from build123d import *

# Parameters (mm, degrees)
ESBO_O1_R                = 60
ESBO_O1_R_2              = 3
RESSALTO_EXTRUS_O4_DEPTH = 30
ESBO_O6_R                = 60
ESBO_O6_R_2              = 5
RESSALTO_EXTRUS_O8_DEPTH = 30
ESBO_O9_R                = 60
CORTE_EXTRUS_O1_DEPTH    = 91
ESBO_O11_W               = 62
ESBO_O11_H               = 15
CORTE_EXTRUS_O2_DEPTH    = 60.514704065
ESBO_O12_R               = 2.5
CORTE_EXTRUS_O3_DEPTH    = 15
ESBO_O15_R               = 3
RESSALTO_EXTRUS_O9_DEPTH = 5
ESBO_O16_R               = 4.75
CORTE_EXTRUS_O4_DEPTH    = 6


with BuildPart() as part:
    # Esboço1 → Ressalto-extrusão4 (new body)
    with BuildSketch(Plane.XY):
        Circle(ESBO_O1_R)
        with Locations((-14.142135624, 14.142135624)):
            Circle(ESBO_O1_R_2, mode=Mode.SUBTRACT)
        with Locations((14.142135624, 14.142135624)):
            Circle(ESBO_O1_R_2, mode=Mode.SUBTRACT)
        with Locations((14.142135624, -14.142135624)):
            Circle(ESBO_O1_R_2, mode=Mode.SUBTRACT)
        with Locations((-14.142135624, -14.142135624)):
            Circle(ESBO_O1_R_2, mode=Mode.SUBTRACT)
        with Locations((0, 20)):
            Circle(ESBO_O1_R_2, mode=Mode.SUBTRACT)
    extrude(amount=-RESSALTO_EXTRUS_O4_DEPTH)

    # Esboço6 → Ressalto-extrusão8 (add)
    with BuildSketch(Plane.XY):
        Circle(ESBO_O6_R)
        with Locations((-14.142135624, -14.142135624)):
            Circle(ESBO_O6_R_2, mode=Mode.SUBTRACT)
        with Locations((14.142135624, -14.142135624)):
            Circle(ESBO_O6_R_2, mode=Mode.SUBTRACT)
        with Locations((-14.142135624, 14.142135624)):
            Circle(ESBO_O6_R_2, mode=Mode.SUBTRACT)
        with Locations((14.142135624, 14.142135624)):
            Circle(ESBO_O6_R_2, mode=Mode.SUBTRACT)
    extrude(amount=-RESSALTO_EXTRUS_O8_DEPTH)

    # Esboço9 → Corte-extrusão1 (cut, through all)
    with BuildSketch(Plane(origin=(0, 0, -30), x_dir=(-1, 0, 0), z_dir=(0, 0, -1))):
        Circle(ESBO_O9_R)
        Polygon((-31, 30), (0, 30), (31, 30), (31, 0), (31, -31), (31, -41), (-31, -41), (-31, -31), (-31, 0), align=None, mode=Mode.SUBTRACT)
    extrude(amount=-CORTE_EXTRUS_O1_DEPTH, mode=Mode.SUBTRACT)

    # Esboço11 → Corte-extrusão2 (cut, through all)
    with BuildSketch(Plane.XY):
        with Locations((0, -33.5)):
            Rectangle(ESBO_O11_W, ESBO_O11_H)
    extrude(amount=-CORTE_EXTRUS_O2_DEPTH, mode=Mode.SUBTRACT)

    # Esboço12 → Corte-extrusão3 (cut)
    with BuildSketch(Plane.XZ.offset(26)):
        with Locations(Location((24.07, -15, 0), (0, 0, 270))):
            Circle(ESBO_O12_R)
        with Locations(Location((0, -15, 0), (0, 0, 270))):
            Circle(ESBO_O12_R)
        with Locations(Location((-24.07, -15, 0), (0, 0, 270))):
            Circle(ESBO_O12_R)
    extrude(amount=-CORTE_EXTRUS_O3_DEPTH, mode=Mode.SUBTRACT)

    # Esboço15 → Ressalto-extrusão9 (add)
    with BuildSketch(Plane.XY):
        with Locations((0, 20)):
            Circle(ESBO_O15_R)
    extrude(amount=RESSALTO_EXTRUS_O9_DEPTH)

    # Esboço16 → Corte-extrusão4 (cut)
    with BuildSketch(Plane(origin=(0, 0, -30), x_dir=(-1, 0, 0), z_dir=(0, 0, -1))):
        with Locations((14.142135624, 14.142135624)):
            Circle(ESBO_O16_R)
        with Locations((14.142135624, -14.142135624)):
            Circle(ESBO_O16_R)
        with Locations((-14.142135624, 14.142135624)):
            Circle(ESBO_O16_R)
        with Locations((-14.142135624, -14.142135624)):
            Circle(ESBO_O16_R)
    extrude(amount=-CORTE_EXTRUS_O4_DEPTH, mode=Mode.SUBTRACT)


solid = part.part
Input: part model. Units: mm. Frame: model coordinates. A direction names the side the tool comes from. Give positions to 0.01 mm unless a question says otherwise; leave off trailing zeros. Loops run counter-clockwise (first coordinate to the right, second up) from the corner with the lowest first, then second, coordinate; pieces in that order, holes last. Notation, with made-up numbers: M -25,41.5 L -5,41.5 A20 ccw -5,65.5 Z; hole C -37,13.5 d8. An arc over 180 degrees is marked long. Use one line per item in the form item = value.
1. Pull-direction query (Z, two-part tool) for faces 1 (the face through (13.2, -17.2, -24)), 2 (the face through (0, 2, 0)), 3 (the face through (-24, -11, -15)), 4 (the face through (9.61, -12.72, -27.04)); classes: released by +Z, released by -Z, zero draft, split by the parting line, or undercut.
Numbers:
face_1 = released by -Z
face_2 = released by +Z
face_3 = undercut
face_4 = zero draft
2. Line query: L1, parallel to X at y = 14, z = -27.5; L2, parallel to Y at x = -11.5, z = -12.5; L3, parallel to Y at x = -10, z = -27.5. Output: solid intervals per line, ascending.
Numbers:
L1 = -31 to -18.89, -9.39 to 9.39, 18.89 to 31
L2 = -26 to -15.56, -12.72 to 12.72, 15.56 to 30
L3 = -26 to -16.47, -11.82 to 11.82, 16.47 to 30
3. Section query D-D, the plane x = -14. Return the cut outline in (y, z), and give its area (3 significant figures).
Numbers:
outline = M -26,-30 L -18.89,-30 L -18.89,-24 L -17.14,-24 L -17.14,0 L -26,0 Z; M -11.15,-24 L -9.39,-24 L -9.39,-30 L 9.39,-30 L 9.39,-24 L 11.15,-24 L 11.15,0 L -11.15,0 Z; M 17.14,-24 L 18.89,-24 L 18.89,-30 L 30,-30 L 30,0 L 17.14,0 Z
area = 1,280 mm²
4. Reachability of faces 5 (the face through (0, 2, -30)), 6 (the face through (-25.591, -18.605, -13.016)), 7 (the face through (-10.64, 17.35, -27.04)) from +Z, -Z, +X, -X, +Y, -Y: full face, straight path, thin tool, end or side. Return the list, or none.
Numbers:
face_5 = -Z, +X, -X, +Y, -Y
face_6 = -Y
face_7 = -Z
5. Section query C-C, the plane z = -9. Return the cut outline in (x, y).
Numbers:
outline = M -31,-26 L 31,-26 L 31,30 L -31,30 Z; hole C -14.14,-14.14 d6; hole C -14.14,14.14 d6; hole C 14.14,-14.14 d6; hole C 14.14,14.14 d6
6. First-contact query: pin 1 (5 mm diameter, centred on x = 14.14, y = 14.14, fed in from -Z); pin 2 (7 mm diameter, centred on x = 14.14, y = -14.14, fed in from -Z); pin 3 (10 mm diameter, centred on x = -2.5, y = -10.5, fed in from +Z). Flat tips, straight axial feed; report the tip coordinate or a pass-through.
Numbers:
pin_1 = through
pin_2 = -24
pin_3 = 0
7. Section query A-A, the plane x = 24.07. Return the cut outline in (y, z).
Numbers:
outline = M -26,-30 L 30,-30 L 30,0 L -26,0 L -26,-12.5 L -11,-12.5 L -11,-17.5 L -26,-17.5 Z
8. Section query B-B, the plane y = 20. Return the cut outline in (x, z).
Numbers:
outline = M -31,-30 L 31,-30 L 31,0 L 3,0 L 3,5 L -3,5 L -3,0 L -31,0 Z
